```python
from build123d import *

# Parameters (mm, degrees)
EXTRUDE_START         = -216.432140614
EXTRUDE_2_DEPTH       = 216.432140614
EXTRUDE_START_2       = -214
EXTRUDE_2_2_OUTLINE_W = 32
EXTRUDE_2_2_OUTLINE_H = 33
EXTRUDE_2_2_DEPTH     = 7.978792001
CUT_EXTRUDE_1_DEPTH   = 220.015687774


with BuildPart() as part:
    # Бобышка-Вытянуть2: read off the stored shape, not the designer's step
    # Бобышка-Вытянуть2 outline → Бобышка-Вытянуть2 (new body)
    with BuildSketch(Plane.XY.offset(EXTRUDE_START)):
        with BuildLine():
            Line((-30, 12), (-30, -12))
            ThreePointArc((-30, -12), (-29.121320344, -14.121320344), (-27, -15))
            Line((-27, -15), (-3, -15))
            ThreePointArc((-3, -15), (-0.878679656, -14.121320344), (0, -12))
            Line((0, -12), (0, 12))
            ThreePointArc((0, 12), (-0.878679656, 14.121320344), (-3, 15))
            Line((-3, 15), (-27, 15))
            ThreePointArc((-27, 15), (-29.121320344, 14.121320344), (-30, 12))
        make_face()
        with BuildLine():
            ThreePointArc((-26, -13), (-27.414213562, -12.414213562), (-28, -11))
            Line((-28, -11), (-28, 11))
            ThreePointArc((-28, 11), (-27.414213562, 12.414213562), (-26, 13))
            Line((-26, 13), (-4, 13))
            ThreePointArc((-4, 13), (-2.585786438, 12.414213562), (-2, 11))
            Line((-2, 11), (-2, -11))
            ThreePointArc((-2, -11), (-2.585786438, -12.414213562), (-4, -13))
            Line((-4, -13), (-26, -13))
        make_face(mode=Mode.SUBTRACT)
    extrude(amount=EXTRUDE_2_DEPTH)

    # Extrude 2 2 outline → Extrude 2 2 (cut)
    with BuildSketch(Plane(origin=(0, 0, 0), x_dir=(1, 0, 0), z_dir=(0, 0.24699838348974407, 0.9690158917961322)).offset(EXTRUDE_START_2)):
        with Locations((-15, 52.5)):
            Rectangle(EXTRUDE_2_2_OUTLINE_W, EXTRUDE_2_2_OUTLINE_H)
    extrude(amount=EXTRUDE_2_2_DEPTH, mode=Mode.SUBTRACT)

    # Эскиз2 → Вырез-Вытянуть1 (cut, through all)
    with BuildSketch(Plane(origin=(0, 0, 0), x_dir=(0, 0, -1), z_dir=(1, 0, 0))):
        Polygon((-3.198950411, 35.913322267), (90.182976942, -15), (69.518016438, -52.902335865), (-23.863910916, -1.989013598), align=None)
    extrude(amount=-CUT_EXTRUDE_1_DEPTH, mode=Mode.SUBTRACT)


solid = part.part
```
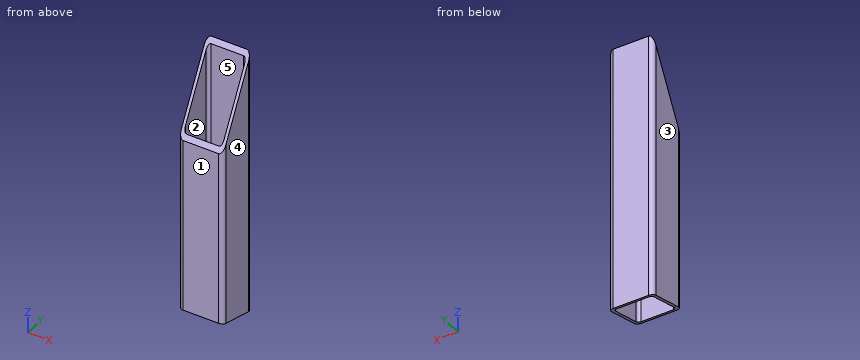
Build history of the part. All positions in model axes, mm. Face numbers are marked on the shaded views. A direction names the side the tool comes from. Coordinates: 2 decimals unless noted, no trailing zeros. Order: outer loops, then holes, each group sorted by start corner. A loop starts at its lowest first (then second) coordinate and runs counter-clockwise, first axis right, second up.
Item 1: Saw through at A-A on x = -6.5. List the corners of the cut face in (y, z).
Filled in:
outline: (-15, -208.79) - (-13, -209.3) - (-13, -86.51) - (-15, -90.18) - close; (13, -215.92) - (15, -216.43) - (15, -35.16) - (13, -38.83) - close
Item 2: Drill centre lines: L1, parallel to X at y = -4, z = -118; L2, parallel to Y at x = -25, z = -111.5; L3, parallel to Y at x = -10, z = -50.5. Where is each one in solid material? Low to high.
Filled in:
L1: x = -30 to -28, -2 to 0
L2: y = -15 to -13, 13 to 15
L3: y = 13 to 15
Item 3: Mould opens along X. For the marked faces 1, 2 and 3 say: released by +X, released by -X, zero draft, split by the parting line, or undercut.
Filled in:
face 1: zero draft
face 2: undercut
face 3: released by -X
Item 4: Saw through at C-C on y = 0.5. List the corners of the cut face in (x, z).
Filled in:
outline: (-30, -212.74) - (-28, -212.74) - (-28, -61.75) - (-30, -61.75) - close; (-2, -212.74) - (0, -212.74) - (0, -61.75) - (-2, -61.75) - close
Item 5: Saw through at B-B on z = -169. List the corners of the cut face in (x, y), then the cut area to 3 significant figures.
Filled in:
outline: (-30, -12) arc R3 ccw to (-27, -15) - (-3, -15) arc R3 ccw to (0, -12) - (0, 12) arc R3 ccw to (-3, 15) - (-27, 15) arc R3 ccw to (-30, 12) - close; hole (-28, -11) arc R2 ccw to (-26, -13) - (-4, -13) arc R2 ccw to (-2, -11) - (-2, 11) arc R2 ccw to (-4, 13) - (-26, 13) arc R2 ccw to (-28, 11) - close
area: 220 mm2
Item 6: Saw through at D-D on z = -64. List the corners of the cut face in (x, y).
Filled in:
outline: (-30, -0.72) - (-28, -0.72) - (-28, 11) arc R2 cw to (-26, 13) - (-4, 13) arc R2 cw to (-2, 11) - (-2, -0.72) - (0, -0.72) - (0, 12) arc R3 ccw to (-3, 15) - (-27, 15) arc R3 ccw to (-30, 12) - close
Item 7: Tool access for the marked faces 4 and 5: list every direction of +Z, -Z, +X, -X, +Y, -Y with a clear straight run to the whole face (end or side of a thin tool).
Filled in:
face 4: +Z, -Z, +X, +Y, -Y
face 5: +Z, -Z
Item 8: Drop flat-ended pins along their axis: pin 1 Ø5 at (x, y) = (-19, 11.5) entering from -Z; pin 2 Ø5 at (x, y) = (-3.5, 2) entering from -Z. Give the stop position or say it passes through.
Filled in:
pin 1: stops at z = -216.18
pin 2: stops at z = -213.63
